Geometry: final body of the model. Coordinates: model frame, mm. Face numbers are marked on the shaded views. Round coordinates to 2 decimals unless told otherwise and drop trailing zeros. Loops run counter-clockwise (first coordinate to the right, second up) from the corner with the lowest first, then second, coordinate; pieces in that order, holes last. Notation, with made-up numbers: (50.5, 60.5) - (91.5, 60.5) arc R21 cw to (91.5, 91.5) - close; hole circle Ø1 at (27.25, 76.25). An arc over 180 degrees is marked (long way). Answer in a Markdown table with one row per item. Add a question column.
Autodesk Inventor part; units mm, degrees
ref_plane "YZ Plane" through (0, 0, 0) normal (1, 0, 0) x (0, 1, 0)
ref_plane "XZ Plane" through (0, 0, 0) normal (0, 1, 0) x (-1, 0, 0)
ref_plane "XY Plane" through (0, 0, 0) normal (0, 0, 1) x (1, 0, 0)
sketch "스케치3" plane through (0, 0, 0) normal (0, 0, 1) x (1, 0, 0)
  line L0 (0, 9) -> (0, -9) construction
  line L1 (-1.5, 9) -> (-1.5, -9)
  line L2 (1.5, -9) -> (1.5, 9)
  arc A0 (1.5, 9) -> (-1.5, 9) centre (0, 9) ccw
  arc A1 (-1.5, -9) -> (1.5, -9) centre (0, -9) ccw
  line L3 (-2.5, 9) -> (-2.5, -9)
  arc A2 (-2.5, -9) -> (2.5, -9) centre (0, -9) ccw
  line L4 (2.5, -9) -> (2.5, 9)
  arc A3 (2.5, 9) -> (-2.5, 9) centre (0, 9) ccw
  line L5 (-3.5, 0) -> (3.5, 0) construction
  line L6 (0, -16.1) -> (0, 16.1) construction
  point P0 (0, 0)
  point P1 (0, 0)
  dimension "d8" = 18
  dimension "d9" = 1.5
  dimension "d10" = 1
  dimension "d11" = 9
extrude "돌출3" add sketch "스케치3" along normal blind 1
sketch "스케치4" plane through (0, 0, 1) normal (0, 0, 1) x (1, 0, 0)
  line L0 (2.5, -9) -> (2.5, 9)
  line L1 (2.5, 2.5) -> (22.5, 2.5)
  line L2 (22.5, 2.5) -> (22.5, -2.5)
  line L3 (22.5, -2.5) -> (2.5, -2.5)
  line L4 (2.5, -2.5) -> (2.5, 2.5)
  point P0 (0, 0)
  point P1 (2.5, -2.5)
  dimension "d14" = 20
  dimension "d15" = 2.5
  dimension "d16" = 5
extrude "돌출4" add sketch "스케치4" against normal blind 1
sketch "스케치5" plane through (0, 0, 1) normal (0, 0, 1) x (1, 0, 0)
  circle A0 centre (20, 0) radius 1
  line L0 (-7.5, 0) -> (27.5, 0) construction
  line L1 (0, -16.1) -> (0, 16.1) construction
  point P0 (0, 0)
  dimension "d19" = 2
  dimension "d20" = 20
extrude "돌출5" add sketch "스케치5" along normal blind 1
mirror "미러1" about plane through (0, 0, 0) normal (1, 0, 0) of "돌출4", "돌출5"
properties part number "축"
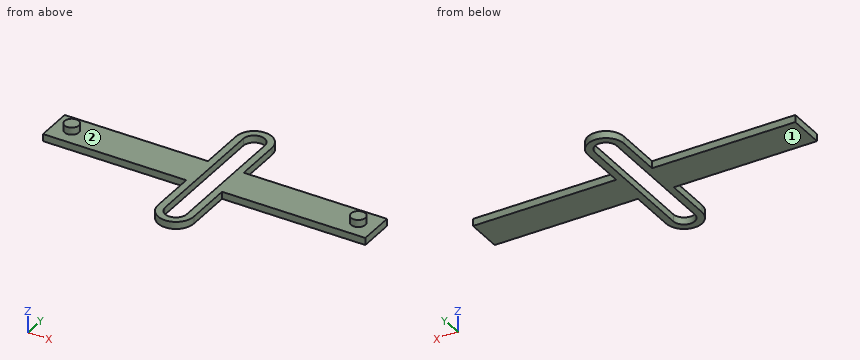
1) Material intervals for line 1 along X through (y, z) = (9, 0.4); line 2 along Z through (x, y) = (8, 1.5); line 3 along Y through (x, z) = (-17.5, 0.35), sorted ascending. Write a range as from..to.
2) Section D-D, the plane y = 9.5. Return the cut outline in (x, z), and give its area (3 significant figures).
3) Section C-C, the plane x = -20. Return the cut outline in (y, z), and give its area (3 significant figures).
4) Contact query for flat-ended pins moving along their axis: pin 1 Ø0.8 at (y, z) = (-5, 0.5) entering from -X; pin 2 Ø1.1 at (y, z) = (-5, 0.5) entering from +X; pin 3 Ø1.1 at (x, z) = (-9.5, 0.5) entering from -Y. Output: stop coordinate, or through.
5) Pull-direction query (X, two-part tool) for the marked faces 1 and 2; classes: pulls with the +X half, pulls with the -X half, needs draft (parallel to the pull), parting line crosses it, or undercut.
6) Section B-B, the plane y = 0. Return the cut outline in (x, z), and give its area (3 significant figures).
7) Section A-A, the plane x = 0. Return the cut outline in (y, z).
Evaluation:
| question | item | result |
|---|---|---|
| 1 | line 1 | x = -2.5..-1.5, 1.5..2.5 |
| 1 | line 2 | z = 0..1 |
| 1 | line 3 | y = -2.5..2.5 |
| 2 | outline | (-2.45, 0) - (-1.41, 0) - (-1.41, 1) - (-2.45, 1) - close; (1.41, 0) - (2.45, 0) - (2.45, 1) - (1.41, 1) - close |
| 2 | area | 2.07 mm² |
| 3 | outline | (-2.5, 0) - (2.5, 0) - (2.5, 1) - (1, 1) - (1, 2) - (-1, 2) - (-1, 1) - (-2.5, 1) - close |
| 3 | area | 7.00 mm² |
| 4 | pin 1 | stops at x = -2.5 |
| 4 | pin 2 | stops at x = 2.5 |
| 4 | pin 3 | stops at y = -2.5 |
| 5 | face 1 | needs draft |
| 5 | face 2 | undercut |
| 6 | outline | (-22.5, 0) - (-1.5, 0) - (-1.5, 1) - (-19, 1) - (-19, 2) - (-21, 2) - (-21, 1) - (-22.5, 1) - close; (1.5, 0) - (22.5, 0) - (22.5, 1) - (21, 1) - (21, 2) - (19, 2) - (19, 1) - (1.5, 1) - close |
| 6 | area | 46.0 mm² |
| 7 | outline | (-11.5, 0) - (-10.5, 0) - (-10.5, 1) - (-11.5, 1) - close; (10.5, 0) - (11.5, 0) - (11.5, 1) - (10.5, 1) - close |
